Geometry check sheet. Reference: the model listing, model coordinates, mm. A direction names the side the tool comes from. Give positions to 0.01 mm unless a question says otherwise; leave off trailing zeros. Write each loop counter-clockwise with the first axis right and the second up, starting at its lowest first coordinate (ties: lowest second). Pieces come first, ordered by that corner, then holes.
(1) Mould release check, pull along X, two halves, no side actions. Record for faces 1 (the flat face through (-5.69, 17.78, -87.83)), 2 (the flat face through (35.4, 0, -81)), 3 (the flat face through (0, 35.4, -81)): +X half, -X half, draft (parallel to the pull), parting line (faces both ways), or undercut.
(2) Tool access check on faces 4 (the flat face through (0, 25.4, -6)), 5 (the flat face through (-5.849, -17.728, -87.833)), 6 (the flat face through (15, 16, -165.1)). Record the directions out of +Z, -Z, +X, -X, +Y, -Y that give a thin tool (end or side, any length) a straight path to the whole face; none if there is none.
(3) Cross-section at C-C (x = -7.5). Record the boundary of the cut face in (y, z).
(4) Thickness scan on line 1 along X through (y, z) = (-17, -10.5); line 2 along X through (y, z) = (0.5, -76). Record the ranges inside material, lowest first.
(5) Cross-section at D-D (y = -23.5). Record the boundary of the cut face in (x, z).
(6) Cross-section at A-A (z = -51). Record the boundary of the cut face in (x, y).
(7) Cross-section at B-B (y = -4.5). Record the boundary of the cut face in (x, z).
```python
from build123d import *

# Parameters (mm, degrees)
F0_W     = 70.8
F0_H     = 70.8
F0_W_2   = 50.8
F0_H_2   = 50.8
F1_DEPTH = 165.1
F2_DEPTH = 12.7
F4_DEPTH = 200.1


with BuildPart() as f1:
    # F0 (on Top) → F1 (new body)
    with BuildSketch(Plane.XY):
        Rectangle(F0_W, F0_H)
        Rectangle(F0_W_2, F0_H_2, mode=Mode.SUBTRACT)
        Rectangle(F0_W_2, F0_H_2)
    extrude(amount=-F1_DEPTH)

    # F0 (on Top) → F2 (cut)
    with BuildSketch(Plane.XY):
        Rectangle(F0_W_2, F0_H_2)
    extrude(amount=-F2_DEPTH, mode=Mode.SUBTRACT)

    # F3 (on face) → F4 (cut)
    with BuildSketch(Plane.XY):
        Polygon((18.667707, -6.065506), (18.667707, 6.065506), (11.537278, 15.8797), (0, 19.628389), (-11.537278, 15.8797), (-18.667707, 6.065506), (-18.667707, -6.065506), (-11.537278, -15.8797), (0, -19.628389), (11.537278, -15.8797), align=None)
    extrude(amount=-F4_DEPTH, mode=Mode.SUBTRACT)


solid = f1.part
```
Reply:
1. face 1: undercut
1. face 2: +X half
1. face 3: draft
2. face 4: +Z
2. face 5: +Z, -Z
2. face 6: -Z, +X, -X, +Y, -Y
3. outline: (-35.4, -165.1) - (-17.19, -165.1) - (-17.19, -12.7) - (-25.4, -12.7) - (-25.4, 0) - (-35.4, 0) - close; (17.19, -165.1) - (35.4, -165.1) - (35.4, 0) - (25.4, 0) - (25.4, -12.7) - (17.19, -12.7) - close
4. line 1: x = -35.4 to -25.4, 25.4 to 35.4
4. line 2: x = -35.4 to -18.67, 18.67 to 35.4
5. outline: (-35.4, -165.1) - (35.4, -165.1) - (35.4, 0) - (25.4, 0) - (25.4, -12.7) - (-25.4, -12.7) - (-25.4, 0) - (-35.4, 0) - close
6. outline: (-35.4, -35.4) - (35.4, -35.4) - (35.4, 35.4) - (-35.4, 35.4) - close; hole (-18.67, -6.07) - (-11.54, -15.88) - (0, -19.63) - (11.54, -15.88) - (18.67, -6.07) - (18.67, 6.07) - (11.54, 15.88) - (0, 19.63) - (-11.54, 15.88) - (-18.67, 6.07) - close
7. outline: (-35.4, -165.1) - (-18.67, -165.1) - (-18.67, -12.7) - (-25.4, -12.7) - (-25.4, 0) - (-35.4, 0) - close; (18.67, -165.1) - (35.4, -165.1) - (35.4, 0) - (25.4, 0) - (25.4, -12.7) - (18.67, -12.7) - close
